CAD build for the part. Positions are in the model's coordinates, mm. Face numbers are marked on the shaded views. Give positions to 0.01 mm unless a question says otherwise; leave off trailing zeros. Write each loop counter-clockwise with the first axis right and the second up, starting at its lowest first coordinate (ties: lowest second). Pieces come first, ordered by that corner, then holes. Notation, with made-up numbers: (41, -10.5) - (85, -10.5) arc R15 ccw to (85, 3.5) - close; hole circle Ø3 at (81.5, -28.75). An arc over 180 degrees is marked (long way). Answer as a JSON object with one key per item and string values.
Autodesk Inventor part; units mm, degrees
ref_plane "YZ Plane" through (0, 0, 0) normal (1, 0, 0) x (0, 1, 0)
ref_plane "XZ Plane" through (0, 0, 0) normal (0, 1, 0) x (-1, 0, 0)
ref_plane "XY Plane" through (0, 0, 0) normal (0, 0, 1) x (1, 0, 0)
sketch "Skizze1" plane through (0, 0, 0) normal (0, 0, 1) x (1, 0, 0)
  circle A0 centre (4.9, 17.1) radius 0.455
  circle A1 centre (4.9, 17.1) radius 0.7
  line L0 (6.3, 15.875) -> (6.3, 17.1)
  line L1 (0, 20) -> (7, 20)
  line L2 (7, 20) -> (7, 18.75)
  line L3 (7, 18.75) -> (1.75, 18.75)
  line L4 (0, 0) -> (9.5856, 0)
  line L5 (0, 20) -> (0, 17.1)
  line L6 (0, 17.1) -> (1.75, 16.75)
  line L7 (1.75, 16.75) -> (4.9, 15)
  line L8 (4.9, 15) -> (6.3, 15.875)
  line L9 (4.9, 15) -> (0, 15) construction
  line L10 (0, 18) -> (0, -3)
  line L11 (-1.9171, 0) -> (11.5027, 0)
  line L12 (4.2, 17.1) -> (1.75, 17.59)
  line L13 (1.75, 17.59) -> (1.75, 18.75)
  line L14 (6.3, 17.1) -> (5.6, 17.1)
  dimension "d0" = 40
  dimension "d1" = 31.75
  dimension "d2" = 1.25
  dimension "d3" = 0.91
  dimension "d4" = 1.4
  dimension "d5" = 30
  dimension "d6" = 33.5
  dimension "d7" = 34.2
  dimension "d8" = 4.9
  dimension "d9" = 6.3
  dimension "d10" = 7
  dimension "d12" = 1.75
revolve "Körper" add sketch "Skizze1" angle 360 about axis through (0, 0, 0) along (1, 0, 0) contours L14 L0 L8 L7 L6 L5 L1 L2 L3 L13 L12 A1
revolve "Feder1" add sketch "Skizze1" angle 360 about axis through (0, 0, 0) along (1, 0, 0) contours A0 | A1
fillet "Rundung1" radius 0.4 3 edges at (7, -20, 0) (1.75, -18.75, 0) (0, -20, 0)
equation "\"d0\" = SD2"
equation "\"d1\" = ABDM"
equation "\"d3\" = SPDI"
equation "\"d4\" = SPDA"
equation "\"d5\" = NND"
equation "\"d6\" = TKDM"
equation "\"d7\" = HLDM"
equation "\"d8\" = SPDST"
equation "\"d9\" = SDI"
equation "\"d10\" = SWDT"
equation "\"d12\" = SD"
equation "\"d11\" = RR"
equation "\"SD2\" = 40"
equation "\"SWDT\" = 7"
equation "\"RR\" = 0.4"
equation "\"SD\" = 1.75"
equation "\"NND\" = 30"
equation "\"SPDA\" = 1.4"
equation "\"SPDI\" = 0.91"
equation "\"TKDM\" = 33.5"
equation "\"HLDM\" = 34.2"
equation "\"ABDM\" = 31.75"
equation "\"SDI\" = 6.3"
equation "\"SPDST\" = 4.9"
equation "\"LAB\" = 0.35"
properties part number "DIN 3760 - A - 30 x 40 x 7 - NBR" material "Gummi"
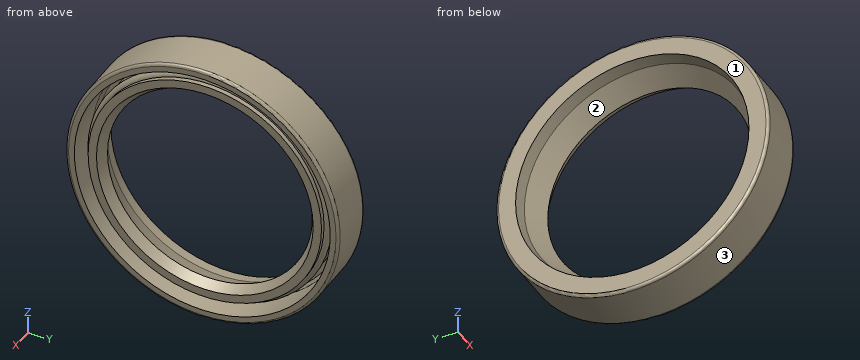
(1) Probe L1, parallel to Y at x = 4.75, z = 4; L2, parallel to Z at x = 6, y = 3.5; L3, parallel to Y at x = 5.5, z = -6. List the from-to ranges inside material, lowest first. Write a range as [from, to].
Answer key:
{"L1": "y = [-19.6, -18.32], [-17.33, -14.54], [14.54, 17.33], [18.32, 19.6]", "L2": "z = [-19.69, -18.42], [-16.74, -15.29], [15.29, 16.74], [18.42, 19.69]", "L3": "y = [-19.08, -17.76], [-16.4, -14.16], [14.16, 16.4], [17.76, 19.08]"}
(2) Flat gauge pins, fed straight in: P1, Ø6, axis at y = 6.5, z = 10.5, coming from the -X side; P2, Ø2, axis at x = 3.5, y = -7.5, coming from the +Z side; P3, Ø3, axis at x = 4, y = 1, coming from the +Z side. Where does each tip first touch, or does it go through?
Answer key:
{"P1": "stops at x = 4.27", "P2": "stops at z = 18.91", "P3": "stops at z = 20"}
(3) Saw through at C-C, the plane x = 3.5. Give the cut face in (y, z).
Answer key:
{"outline": "circle Ø40 at (0, 0); circle Ø34.48 at (0, 0); hole circle Ø37.5 at (0, 0); hole circle Ø31.56 at (0, 0)"}
(4) Pull direction Y, two halves, no side cores. Call the marked faces 1, 2 and 3: pulls with the +Y half, pulls with the -Y half, needs draft (parallel to the pull), parting line crosses it, or undercut.
Answer key:
{"face 1": "needs draft", "face 2": "undercut", "face 3": "parting line crosses it"}
